```python
from build123d import *

# Parameters (mm, degrees)
BOSS_EXTRUDE1_DEPTH     = 1.524
BOSS_EXTRUDE2_START     = -15.875
BOSS_EXTRUDE2_OUTLINE_R = 2.413
BOSS_EXTRUDE2_DEPTH     = 15.875
CUT_EXTRUDE1_DEPTH      = 162.377710637
CUT_EXTRUDE2_DEPTH      = 162.267022773


# Read off the part's stored shape, not the designer's step: Boss-Extrude2
with BuildPart() as part:
    # Sketch1 → Boss-Extrude1 (new body)
    with BuildSketch(Plane(origin=(0, 0, 0), x_dir=(1, 0, 0), z_dir=(0, 1, 0))):
        Polygon((-101.6, -7.9375), (-160.698602846, -7.9375), (-160.698602846, 7.9375), (-101.6, 7.9375), (101.6, 7.9375), (101.6, -7.9375), align=None)
    extrude(amount=BOSS_EXTRUDE1_DEPTH)

    # Boss-Extrude2 outline → Boss-Extrude2 (add)
    with BuildSketch(Plane.XY.offset(7.9375).offset(BOSS_EXTRUDE2_START)):
        with BuildLine():
            add(Edge.make_bspline(
                [(107.228546138, 6.692607406), (106.366027923, 7.18125968), (105.140033894, 7.42790314), (103.583408394, 7.287922485), (101.756786703, 6.577932625), (99.786331846, 5.041015057)],
                knots=[0, 0, 0, 0, 0, 0, 1, 1, 1, 1, 1, 1], degree=5))
            ThreePointArc((107.228546138, 6.692607406), (108.258782429, 4.761783473), (107.30453503, 2.792296286))
            add(Edge.make_bspline(
                [(101.6, 1.524), (103.258114517, 1.448306251), (104.638933259, 1.583946831), (105.766741539, 1.881154947), (106.652889556, 2.297992507), (107.30453503, 2.792296286)],
                knots=[0, 0, 0, 0, 0, 0, 1, 1, 1, 1, 1, 1], degree=5))
            Line((101.6, 1.524), (101.6, 0))
            add(Edge.make_bspline(
                [(101.6, 0), (104.748480566, -0.003746591), (109.050367624, 0.259943099), (110.73800353, 3.235869603), (109.946934459, 5.044027479), (108.94689031, 7.25796652)],
                knots=[0, 0, 0, 0, 0, 0, 1, 1, 1, 1, 1, 1], degree=5))
            add(Edge.make_bspline(
                [(108.94689031, 7.25796652), (106.455515071, 10.263008134), (101.235622898, 14.016404122), (98.534099755, 12.238404022), (96.99562172, 12.065011937)],
                knots=[0, 0, 0, 0, 0, 1, 1, 1, 1, 1], degree=4))
            ThreePointArc((96.99562172, 12.065011937), (93.706192437, 6.691697876), (99.786331846, 5.041015057))
        make_face()
        with Locations((97.364988112, 8.145377073)):
            Circle(BOSS_EXTRUDE2_OUTLINE_R, mode=Mode.SUBTRACT)
    extrude(amount=BOSS_EXTRUDE2_DEPTH)

    # Sketch6 → Cut-Extrude1 (cut, through all)
    with BuildSketch(Plane.XZ):
        Polygon((109.757786654, 7.9375), (101.6, 7.9375), (101.6, 6.972022749), (109.757786654, 5.238031667), align=None)
        Polygon((109.757786654, -5.238031667), (101.6, -6.972022749), (101.6, -7.9375), (109.757786654, -7.9375), align=None)
        Polygon((101.6, 7.9375), (97.057786654, 7.9375), (101.6, 6.972022749), align=None)
        Polygon((101.6, -7.9375), (101.6, -6.972022749), (97.057786654, -7.9375), align=None)
    extrude(amount=-CUT_EXTRUDE1_DEPTH, mode=Mode.SUBTRACT)

    # Sketch7 → Cut-Extrude2 (cut, through all)
    with BuildSketch(Plane(origin=(0, 1.524, 0), x_dir=(1, 0, 0), z_dir=(0, 1, 0))):
        Polygon((101.6, 5.759486397), (107.30453503, 5.759486397), (107.30453503, 11.866720982), (85.552872932, 11.866720982), (85.552872932, 7.9375), (97.057786654, 7.9375), (101.6, 6.972022749), align=None)
        Polygon((85.552872932, 5.759486397), (101.6, 5.759486397), (101.6, 6.972022749), (97.057786654, 7.9375), (85.552872932, 7.9375), align=None)
        Polygon((101.6, -6.972022749), (101.6, -5.759486397), (85.552872932, -5.759486397), (85.552872932, -7.9375), (97.057786654, -7.9375), align=None)
        Polygon((107.30453503, -7.9375), (107.30453503, -5.759486397), (101.6, -5.759486397), (101.6, -6.972022749), (97.057786654, -7.9375), align=None)
    extrude(amount=CUT_EXTRUDE2_DEPTH, mode=Mode.SUBTRACT)


solid = part.part
```
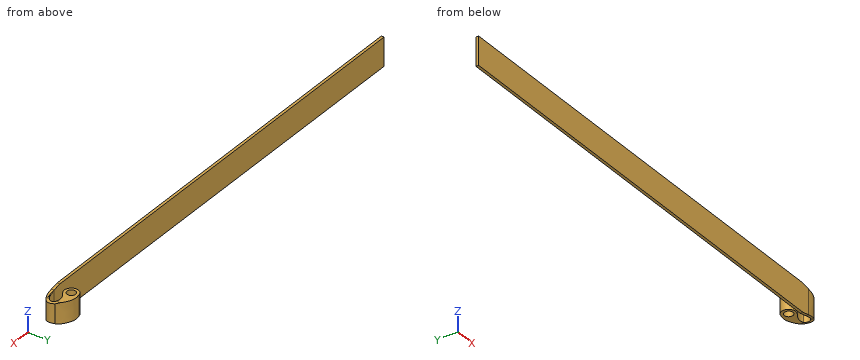
CAD build for the part. Positions are in the model's coordinates, mm. Coordinates: 2 decimals unless noted, no trailing zeros. Order: outer loops, then holes, each group sorted by start corner. A loop starts at its lowest first (then second) coordinate and runs counter-clockwise, first axis right, second up.
(1) Saw through at A-A, the plane x = -122.5. Write the cut outline in (y, z).
Solution:
outline: (0, -7.94) - (1.52, -7.94) - (1.52, 7.94) - (0, 7.94) - close
(2) Pin check, flat tips, straight feed: pin 1 Ø4 at (y, z) = (4, 4) entering from +X; pin 2 Ø1.5 at (x, z) = (35, -5.5) entering from +Y; pin 3 Ø5 at (x, y) = (-7.5, 6) entering from -Z; pin 4 Ø4 at (x, y) = (102, 7) entering from -Z. Stop position of each tip, or through.
Solution:
pin 1: stops at x = 109.76
pin 2: stops at y = 1.52
pin 3: passes through
pin 4: stops at z = -5.76
(3) Drill centre lines: L1, parallel to X at y = 8, z = -1.5; L2, parallel to Y at x = 28, z = 2; L3, parallel to X at y = 9.5, z = 3. Where is each one in solid material? Low to high.
Solution:
L1: x = 93.43 to 94.96, 99.77 to 108.29
L2: y = 0 to 1.52
L3: x = 93.67 to 95.37, 99.36 to 106.66
